```python
from build123d import *

# Parameters (mm, degrees)
SKETCH1_W           = 56
SKETCH1_H           = 56
BOSS_EXTRUDE1_DEPTH = 46
SKETCH2_R           = 22.5
CUT_EXTRUDE1_DEPTH  = 3
SKETCH3_R           = 11.5
CUT_EXTRUDE2_DEPTH  = 50
SKETCH4_R           = 2.5
CUT_EXTRUDE3_DEPTH  = 10
CUT_EXTRUDE4_DEPTH  = 36
SKETCH6_W           = 34.5
SKETCH6_H           = 15
BOSS_EXTRUDE2_DEPTH = 30
SKETCH7_R           = 2.15
CUT_EXTRUDE5_DEPTH  = 30
FILLET1_R           = 3
SKETCH8_R           = 3.5
CUT_EXTRUDE6_DEPTH  = 4
CIRPATTERN2_COUNT   = 4
FILLET2_R           = 3
FILLET3_R           = 3
FILLET4_R           = 3
FILLET5_R           = 3


with BuildPart() as part:
    # Sketch1 → Boss-Extrude1 (new body)
    with BuildSketch(Plane(origin=(0, 0, 0), x_dir=(1, 0, 0), z_dir=(0, 1, 0))):
        Rectangle(SKETCH1_W, SKETCH1_H)
    extrude(amount=BOSS_EXTRUDE1_DEPTH)

    # Sketch2 → Cut-Extrude1 (cut)
    with BuildSketch(Plane(origin=(0, 46, 0), x_dir=(1, 0, 0), z_dir=(0, 1, 0))):
        with Locations(Location((0, 0, 0), (0, 0, 270))):
            Circle(SKETCH2_R)
    extrude(amount=-CUT_EXTRUDE1_DEPTH, mode=Mode.SUBTRACT)

    # Sketch3 → Cut-Extrude2 (cut)
    with BuildSketch(Plane(origin=(0, 43, 0), x_dir=(1, 0, 0), z_dir=(0, 1, 0))):
        with Locations(Location((0, 0, 0), (0, 0, 270))):
            Circle(SKETCH3_R)
    extrude(amount=-CUT_EXTRUDE2_DEPTH, mode=Mode.SUBTRACT)

    # Sketch4 → Cut-Extrude3 (cut)
    with BuildSketch(Plane(origin=(0, 46, 0), x_dir=(1, 0, 0), z_dir=(0, 1, 0))):
        with Locations(Location((-22, 22, 0), (0, 0, 270))):
            Circle(SKETCH4_R)
        with Locations(Location((22, 22, 0), (0, 0, 90))):
            Circle(SKETCH4_R)
        with Locations(Location((22, -22, 0), (0, 0, 270))):
            Circle(SKETCH4_R)
        with Locations(Location((-22, -22, 0), (0, 0, 90))):
            Circle(SKETCH4_R)
    extrude(amount=-CUT_EXTRUDE3_DEPTH, mode=Mode.SUBTRACT)

    # Sketch5 → Cut-Extrude4 (cut)
    with BuildSketch(Plane.XZ):
        with BuildLine():
            Line((-22, 17.25), (-28, 17.25))
            Line((-28, 17.25), (-28, 28))
            Line((-28, 28), (-17.25, 28))
            Line((-17.25, 28), (-17.25, 22))
            ThreePointArc((-17.25, 22), (-18.641242789, 18.641242789), (-22, 17.25))
        make_face()
        with BuildLine():
            Line((17.25, 22), (17.25, 28))
            Line((17.25, 28), (28, 28))
            Line((28, 28), (28, 17.25))
            Line((28, 17.25), (22, 17.25))
            ThreePointArc((22, 17.25), (18.641242789, 18.641242789), (17.25, 22))
        make_face()
        with BuildLine():
            Line((-28, -17.25), (-28, -28))
            Line((-28, -28), (-17.25, -28))
            Line((-17.25, -28), (-17.25, -22))
            ThreePointArc((-17.25, -22), (-18.641242789, -18.641242789), (-22, -17.25))
            Line((-22, -17.25), (-28, -17.25))
        make_face()
        with BuildLine():
            Line((22, -17.25), (28, -17.25))
            Line((28, -17.25), (28, -28))
            Line((28, -28), (17.25, -28))
            Line((17.25, -28), (17.25, -22))
            ThreePointArc((17.25, -22), (18.641242789, -18.641242789), (22, -17.25))
        make_face()
    extrude(amount=-CUT_EXTRUDE4_DEPTH, mode=Mode.SUBTRACT)

    # Sketch6 → Boss-Extrude2 (add)
    with BuildSketch(Plane(origin=(0, 0, -28), x_dir=(-1, 0, 0), z_dir=(0, 0, -1))):
        with Locations((0, 7.5)):
            Rectangle(SKETCH6_W, SKETCH6_H)
    boss_extrude2 = extrude(amount=BOSS_EXTRUDE2_DEPTH)

    # Sketch7 → Cut-Extrude5 (cut)
    with BuildSketch(Plane(origin=(0, 15, 0), x_dir=(1, 0, 0), z_dir=(0, 1, 0))):
        with Locations(Location((-10.25, 51, 0), (0, 0, 270))):
            Circle(SKETCH7_R)
        with Locations(Location((10.25, 51, 0), (0, 0, 90))):
            Circle(SKETCH7_R)
        with Locations(Location((10.25, 35, 0), (0, 0, 270))):
            Circle(SKETCH7_R)
        with Locations(Location((-10.25, 35, 0), (0, 0, 90))):
            Circle(SKETCH7_R)
    cut_extrude5 = extrude(amount=-CUT_EXTRUDE5_DEPTH, mode=Mode.SUBTRACT)

    # Fillet1
    fillet1_edges = [part.edges().sort_by_distance(p)[0] for p in [
        (0, 15, -28),
    ]]
    fillet(fillet1_edges, radius=FILLET1_R)

    # Sketch8 → Cut-Extrude6 (cut)
    with BuildSketch(Plane(origin=(0, 15, 0), x_dir=(1, 0, 0), z_dir=(0, 1, 0))):
        with Locations(Location((-10.25, 51, 0), (0, 0, 270))):
            Circle(SKETCH8_R)
        with Locations(Location((10.25, 51, 0), (0, 0, 270))):
            Circle(SKETCH8_R)
        with Locations(Location((-10.25, 35, 0), (0, 0, 270))):
            Circle(SKETCH8_R)
        with Locations(Location((10.25, 35, 0), (0, 0, 270))):
            Circle(SKETCH8_R)
    cut_extrude6 = extrude(amount=-CUT_EXTRUDE6_DEPTH, mode=Mode.SUBTRACT)

    # CirPattern2: Boss-Extrude2, Cut-Extrude5, Cut-Extrude6 ×4 about axis
    cirpattern2_axis = Axis((0, 0, 0), (0, 1, 0))
    add([boss_extrude2.rotate(cirpattern2_axis, i * 360 / CIRPATTERN2_COUNT) for i in range(1, CIRPATTERN2_COUNT)])
    add([cut_extrude5.rotate(cirpattern2_axis, i * 360 / CIRPATTERN2_COUNT) for i in range(1, CIRPATTERN2_COUNT)], mode=Mode.SUBTRACT)
    add([cut_extrude6.rotate(cirpattern2_axis, i * 360 / CIRPATTERN2_COUNT) for i in range(1, CIRPATTERN2_COUNT)], mode=Mode.SUBTRACT)

    # Fillet2
    fillet2_edges = [part.edges().sort_by_distance(p)[0] for p in [
        (-28, 15, 0),
        (0, 15, 28),
        (28, 15, 0),
    ]]
    fillet(fillet2_edges, radius=FILLET2_R)

    # Fillet3
    fillet3_edges = [part.edges().sort_by_distance(p)[0] for p in [
        (17.25, 7.5, -58),
        (-17.25, 7.5, -58),
        (-58, 7.5, -17.25),
        (-58, 7.5, 17.25),
        (-17.25, 7.5, 58),
        (17.25, 7.5, 58),
        (58, 7.5, 17.25),
        (58, 7.5, -17.25),
    ]]
    fillet(fillet3_edges, radius=FILLET3_R)

    # Fillet4
    fillet4_edges = [part.edges().sort_by_distance(p)[0] for p in [
        (17.25, 15.878679656, -28.878679656),
        (-17.25, 15.878679656, -28.878679656),
        (28.878679656, 15.878679656, 17.25),
        (28.878679656, 15.878679656, -17.25),
        (-28.878679656, 15.878679656, -17.25),
        (-28.878679656, 15.878679656, 17.25),
        (0, 15, -58),
        (17.25, 15, -43),
        (-17.25, 15, -43),
        (-16.371320344, 15, -57.121320344),
        (16.371320344, 15, -57.121320344),
        (58, 15, 0),
        (43, 15, -17.25),
        (43, 15, 17.25),
        (57.121320344, 15, 16.371320344),
        (57.121320344, 15, -16.371320344),
        (-58, 15, 0),
        (-43, 15, 17.25),
        (-43, 15, -17.25),
        (-57.121320344, 15, -16.371320344),
        (-57.121320344, 15, 16.371320344),
        (28, 27, 17.25),
        (-28, 27, -17.25),
        (-17.25, 27, -28),
        (28, 27, -17.25),
        (17.25, 27, -28),
        (28, 41, 28),
        (-28, 41, 28),
        (-28, 41, -28),
        (28, 41, -28),
        (-28, 27, 17.25),
    ]]
    fillet(fillet4_edges, radius=FILLET4_R)

    # Fillet5
    fillet5_edges = [part.edges().sort_by_distance(p)[0] for p in [
        (-17.25, 15.878679656, 28.878679656),
        (17.25, 15.878679656, 28.878679656),
        (0, 15, 58),
        (17.25, 15, 43),
        (-17.25, 15, 43),
        (-16.371320344, 15, 57.121320344),
        (16.371320344, 15, 57.121320344),
        (17.25, 27, 28),
        (-17.25, 27, 28),
    ]]
    fillet(fillet5_edges, radius=FILLET5_R)


solid = part.part
```
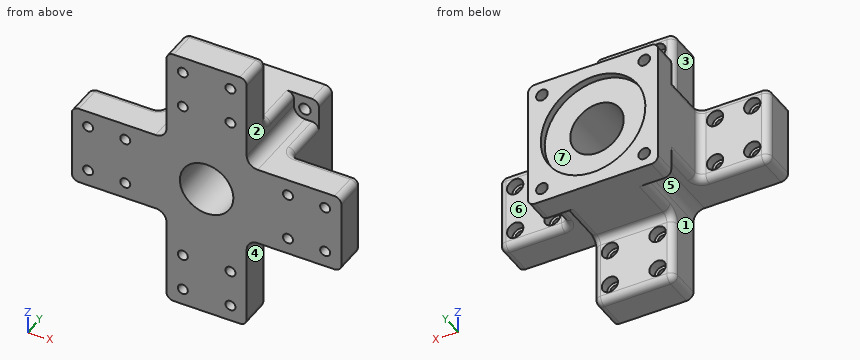
The model under review builds one solid part; all positions refer to its coordinate system, in mm. Face numbers are marked on the shaded views. A direction names the side the tool comes from. Give positions to 0.01 mm unless a question says otherwise; leave off trailing zeros. Loops run counter-clockwise (first coordinate to the right, second up) from the corner with the lowest first, then second, coordinate; pieces in that order, holes last. Notation, with made-up numbers: (43.25, 27.5) - (102.25, 27.5) arc R16 cw to (102.25, 36.5) - close; hole circle Ø10 at (-26.75, 80). An arc over 180 degrees is marked (long way). Answer as a JSON object with one key per item and string values.
Q1. Add section C-C on y = 21. State the section outline as (x, z) points, plus the area to 3 significant figures.
Worked out:
{"outline": "(-28, -14.25) arc R3 ccw to (-25, -17.25) - (-22, -17.25) arc R4.75 cw to (-17.25, -22) - (-17.25, -25) arc R3 ccw to (-14.25, -28) - (14.25, -28) arc R3 ccw to (17.25, -25) - (17.25, -22) arc R4.75 cw to (22, -17.25) - (25, -17.25) arc R3 ccw to (28, -14.25) - (28, 14.25) arc R3 ccw to (25, 17.25) - (22, 17.25) arc R4.75 cw to (17.25, 22) - (17.25, 25) arc R3 ccw to (14.25, 28) - (-14.25, 28) arc R3 ccw to (-17.25, 25) - (-17.25, 22) arc R4.75 cw to (-22, 17.25) - (-25, 17.25) arc R3 ccw to (-28, 14.25) - close; hole circle Ø23 at (0, 0)", "area": "2,260 mm^2"}
Q2. Add section A-A on x = 0. State the section outline as (y, z) points.
Worked out:
{"outline": "(0, -58) - (12, -58) arc R3 ccw to (15, -55) - (15, -31) arc R3 cw to (18, -28) - (46, -28) - (46, -22.5) - (43, -22.5) - (43, -11.5) - (0, -11.5) - close; (0, 11.5) - (43, 11.5) - (43, 22.5) - (46, 22.5) - (46, 28) - (18, 28) arc R3 cw to (15, 31) - (15, 55) arc R3 ccw to (12, 58) - (0, 58) - close"}
Q3. Mouldability with a two-part tool opening along Z and no side actions: class the marked faces 5, 6 and 7 as +Z half, -Z half, draft (parallel to the pull), parting line (faces both ways), or undercut.
Worked out:
{"face 5": "-Z half", "face 6": "draft", "face 7": "undercut"}
Q4. Insertion check: pin 1 (16.5 mm diameter, centred on x = -41, y = 9.5, fed in from -Z); pin 2 (5 mm diameter, centred on x = -51, z = -10.25, fed in from +Y); pin 3 (1.5 mm diameter, centred on x = 27.5, y = 5.5, fed in from +Z). Each pin has a flat end and moves straight along its axis. Give the tip position at first contact, or say it passes through.
Worked out:
{"pin 1": "stops at z = -17.25", "pin 2": "stops at y = 11", "pin 3": "stops at z = 17.25"}
Q5. Add section D-D on x = 35. State the section outline as (y, z) points, plus the area to 3 significant figures.
Worked out:
{"outline": "(0, -17.25) - (12, -17.25) arc R3 ccw to (15, -14.25) - (15, -13.75) - (11, -13.75) - (11, -12.4) - (0, -12.4) - close; (0, -8.1) - (11, -8.1) - (11, -6.75) - (15, -6.75) - (15, 6.75) - (11, 6.75) - (11, 8.1) - (0, 8.1) - close; (0, 12.4) - (11, 12.4) - (11, 13.75) - (15, 13.75) - (15, 14.25) arc R3 ccw to (12, 17.25) - (0, 17.25) - close", "area": "363 mm^2"}
Q6. For the marked faces 1, 2, 3 and 4, list the 3-axis set-ups (+Z, -Z, +X, -X, +Y, -Y) from which the entire face can be reached by the end or side of a thin tool; tool diameter is ignored.
Worked out:
{"face 1": "-Z, -X, -Y", "face 2": "+Z, +X, -Y", "face 3": "+Z, -X, -Y", "face 4": "-Z, +X, -Y"}
Q7. To check wall thickness, follow line 1 along X through (y, z) = (41, 0); line 2 along X through (y, z) = (11, 0); line 3 along Y through (x, z) = (-10, -9.5). State the ranges of each line that lie inside material, in increasing order.
Worked out:
{"line 1": "x = -28 to -11.5, 11.5 to 28", "line 2": "x = -58 to -11.5, 11.5 to 58", "line 3": "y = 0 to 43"}
Q8. Add section B-B on z = -51. State the section outline as (x, y) points.
Worked out:
{"outline": "(-17.25, 0) - (-12.4, 0) - (-12.4, 11) - (-13.75, 11) - (-13.75, 15) - (-14.25, 15) arc R3 ccw to (-17.25, 12) - close; (-8.1, 0) - (8.1, 0) - (8.1, 11) - (6.75, 11) - (6.75, 15) - (-6.75, 15) - (-6.75, 11) - (-8.1, 11) - close; (12.4, 0) - (17.25, 0) - (17.25, 12) arc R3 ccw to (14.25, 15) - (13.75, 15) - (13.75, 11) - (12.4, 11) - close"}
